from build123d import *

# Parameters (mm, degrees)
SKETCH_1_R      = 1.6
EXTRUDE_1_DEPTH = 6


with BuildPart() as part:
    # 草图1 → 凸台-拉伸1 (new, symmetric)
    with BuildSketch(Plane.XY):
        Polygon((11.5, 0), (11.5, 18), (16, 18), (16, 23), (11.5, 23), (11.5, 29), (2.5, 29), (2.5, 34), (-2.5, 34), (-2.5, 29), (-11.5, 29), (-11.5, 23), (-16, 23), (-16, 18), (-11.5, 18), (-11.5, 0), align=None)
        with Locations((14, 20.5)):
            Circle(SKETCH_1_R, mode=Mode.SUBTRACT)
        with Locations((-14, 20.5)):
            Circle(SKETCH_1_R, mode=Mode.SUBTRACT)
    extrude(amount=EXTRUDE_1_DEPTH, both=True)


solid = part.part
For this review, take the finished solid that the model builds, in its own axes (mm). A direction names the side the tool comes from. Round coordinates to 2 decimals unless told otherwise and drop trailing zeros. Loops run counter-clockwise (first coordinate to the right, second up) from the corner with the lowest first, then second, coordinate; pieces in that order, holes last. Notation, with made-up numbers: (-3.5, 20.5) - (49.5, 20.5) arc R18 cw to (49.5, 46.5) - close; hole circle Ø2 at (53.25, 36). An arc over 180 degrees is marked (long way). Answer as CSV lines item,"result".
(1) Wall thickness on line 1 (Y direction, x = 14, z = 2.25); line 2 (Y direction, x = 7, z = 0.25); line 3 (X direction, y = 14.5, z = -0.25): over which ranges is each line inside the solid? List them lowest first.
Checked values:
line 1,"y = 18 to 18.9, 22.1 to 23"
line 2,"y = 0 to 29"
line 3,"x = -11.5 to 11.5"
(2) Consider section B-B on x = 14. Give the boundary of the cut face in (y, z), then the cut area to 3 significant figures.
Checked values:
outline,"(18, -6) - (18.9, -6) - (18.9, 6) - (18, 6) - close; (22.1, -6) - (23, -6) - (23, 6) - (22.1, 6) - close"
area,"21.6 mm2"
(3) Consider section D-D on x = -4. Give the boundary of the cut face in (y, z), then the cut area to 3 significant figures.
Checked values:
outline,"(0, -6) - (29, -6) - (29, 6) - (0, 6) - close"
area,"348 mm2"
(4) Consider section C-C on z = -3.25. Give the boundary of the cut face in (x, y).
Checked values:
outline,"(-16, 18) - (-11.5, 18) - (-11.5, 0) - (11.5, 0) - (11.5, 18) - (16, 18) - (16, 23) - (11.5, 23) - (11.5, 29) - (2.5, 29) - (2.5, 34) - (-2.5, 34) - (-2.5, 29) - (-11.5, 29) - (-11.5, 23) - (-16, 23) - close; hole circle Ø3.2 at (-14, 20.5); hole circle Ø3.2 at (14, 20.5)"
(5) Insertion check: P1, Ø1.3, axis at x = -14.5, z = -3, coming from the +Y side; P2, Ø1.8, axis at y = 26.5, z = -0.5, coming from the -X side; P3, Ø5.5, axis at y = 32.5, z = 0, coming from the -X side. Each pin has a flat end and moves straight along its axis. Give the tip position at first contact, or say it passes through.
Checked values:
P1,"stops at y = 23"
P2,"stops at x = -11.5"
P3,"stops at x = -2.5"
(6) Consider section A-A on y = 20.5. Give the boundary of the cut face in (x, z).
Checked values:
outline,"(-16, -6) - (-15.6, -6) - (-15.6, 6) - (-16, 6) - close; (-12.4, -6) - (12.4, -6) - (12.4, 6) - (-12.4, 6) - close; (15.6, -6) - (16, -6) - (16, 6) - (15.6, 6) - close"
(7) Mouldability with a two-part tool opening along Y and no side actions: class faces 5 (the face through (-14, 18, 0)), 6 (the face through (2.5, 31, 0)), 7 (the face through (12.82, 21.58, -0.08)) as +Y half, -Y half, draft (parallel to the pull), parting line (faces both ways), or undercut.
Checked values:
face 5,"-Y half"
face 6,"draft"
face 7,"undercut"
(8) Tool access review of faces 1 (the face through (14, 18, 0)), 2 (the face through (14, 23, 0)), 3 (the face through (-2.5, 32, 0)), 4 (the face through (-11.5, 9, 0)): name each direction out of +Z, -Z, +X, -X, +Y, -Y from which nothing blocks a thin tool from reaching the whole face with its end or side.
Checked values:
face 1,"+Z, -Z, +X, -Y"
face 2,"+Z, -Z, +X, +Y"
face 3,"+Z, -Z, -X, +Y"
face 4,"+Z, -Z, -X, -Y"
